from build123d import *

# Parameters (mm, degrees)
SKETCH1_R           = 5.78131598
BOSS_EXTRUDE1_DEPTH = 12.7
SKETCH2_W           = 12.7
SKETCH2_H           = 6.35
CUT_EXTRUDE1_DEPTH  = 33.528


with BuildPart() as part:
    # Sketch1 → Boss-Extrude1 (new body)
    with BuildSketch(Plane(origin=(0, 0, 0), x_dir=(1, 0, 0), z_dir=(0, 1, 0))):
        with BuildLine():
            Line((-36.7158591, 9.525), (-62.1158591, 9.525))
            Line((-62.1158591, 9.525), (-62.1158591, 28.575))
            ThreePointArc((-62.1158591, 28.575), (-49.4158591, 41.275), (-36.7158591, 28.575))
            Line((-36.7158591, 28.575), (-36.7158591, 9.525))
        make_face()
        with Locations(Location((-49.4158591, 28.575, 0), (0, 0, 270))):
            Circle(SKETCH1_R, mode=Mode.SUBTRACT)
    extrude(amount=BOSS_EXTRUDE1_DEPTH)

    # Sketch2 → Cut-Extrude1 (cut)
    with BuildSketch(Plane(origin=(-36.7158591, 0, 0), x_dir=(0, 0, -1), z_dir=(1, 0, 0))):
        with Locations((34.925, 6.35)):
            Rectangle(SKETCH2_W, SKETCH2_H)
        Polygon((28.575, 9.525), (12.7, 9.525), (12.7, 6.35), (12.7, 3.175), (28.575, 3.175), align=None)
    extrude(amount=-CUT_EXTRUDE1_DEPTH, mode=Mode.SUBTRACT)


solid = part.part
Part model, mm, in its own coordinate system. A direction names the side the tool comes from. Give positions to 0.01 mm unless a question says otherwise; leave off trailing zeros. Loops run counter-clockwise (first coordinate to the right, second up) from the corner with the lowest first, then second, coordinate; pieces in that order, holes last. Notation, with made-up numbers: (28, 66.5) -> (72, 66.5) arc R21 cw to (72, 80.5) -> close; hole circle Ø6 at (-6.5, 74.5). An arc over 180 degrees is marked (long way). Write each question's results on one line, items separated by ' | '. Start each with the question number.
Q1. Pull direction X, two halves, no side cores. Call faces 1 (the face through (-47.68, 1.57, -23.06)), 2 (the face through (-62.116, 2, -17)), 3 (the face through (-49, 6, -12.7)): +X half, -X half, draft (parallel to the pull), parting line (faces both ways), or undercut.
Q2. Band-saw the part on C-C on x = -53. List the corners of the cut face in (y, z) (3 decimals).
Q3. Wall check: L1, parallel to Y at x = -40.75, z = -23.5 (3 decimals); L2, parallel to Z at x = -38.5, y = 5.75 (3 decimals); L3, parallel to X at y = 10.5, z = -32.5. Give the ranges that are in metal, low to high.
Q4. Band-saw the part on D-D on y = 11. List the corners of the cut face in (x, z) (3 decimals), plus the area to 3 significant figures.
Q5. Band-saw the part on B-B on z = -24. List the corners of the cut face in (x, y) (3 decimals), plus the area to 3 significant figures.
Q6. Pin check, flat tips, straight feed: P1, Ø10, axis at x = -57, z = -24.5, coming from the -Y side; P2, Ø1.5, axis at x = -49, y = 6, coming from the -Z side; P3, Ø2, axis at y = 6, z = -19, coming from the +X side; P4, Ø2, axis at y = 1.5, z = -34.5, coming from the -X side. Stop position of each tip, or through.
Q7. Band-saw the part on A-A on z = -18.5. List the corners of the cut face in (x, y) (3 decimals), plus the area to 3 significant figures.
Q8. Which spindle directions (+Z, -Z, +X, -X, +Y, -Y) get a long thin tool onto all of the face, cutting with end or side? Do faces 4 (the face through (-49, 9.525, -21)), 5 (the face through (-49.7, 11.09, -41.27)). Say none if no direction does.
Results are:
1) face 1: undercut | face 2: -X half | face 3: draft
2) outline: (0, -40.759) -> (3.175, -40.759) -> (3.175, -33.111) -> (0, -33.111) -> close; (0, -24.039) -> (3.175, -24.039) -> (3.175, -12.7) -> (9.525, -12.7) -> (9.525, -24.039) -> (12.7, -24.039) -> (12.7, -9.525) -> (0, -9.525) -> close; (9.525, -40.759) -> (12.7, -40.759) -> (12.7, -33.111) -> (9.525, -33.111) -> close
3) L1: y = 0 to 3.175, 9.525 to 12.7 | L2: z = -12.7 to -9.525 | L3: x = -61.49 to -53.66, -45.17 to -37.34
4) outline: (-62.116, -28.575) arc R12.7 ccw to (-36.716, -28.575) -> (-36.716, -9.525) -> (-62.116, -9.525) -> close; hole circle Ø11.563 at (-49.416, -28.575) | area: 632 mm²
5) outline: (-62.116, 0) -> (-52.95, 0) -> (-52.95, 3.175) -> (-62.116, 3.175) -> close; (-62.116, 9.525) -> (-52.95, 9.525) -> (-52.95, 12.7) -> (-62.116, 12.7) -> close; (-45.881, 0) -> (-36.716, 0) -> (-36.716, 3.175) -> (-45.881, 3.175) -> close; (-45.881, 9.525) -> (-36.716, 9.525) -> (-36.716, 12.7) -> (-45.881, 12.7) -> close | area: 116 mm²
6) P1: stops at y = 0 | P2: stops at z = -12.7 | P3: passes through | P4: stops at x = -61.12
7) outline: (-62.116, 0) -> (-36.716, 0) -> (-36.716, 3.175) -> (-62.116, 3.175) -> close; (-62.116, 9.525) -> (-36.716, 9.525) -> (-36.716, 12.7) -> (-62.116, 12.7) -> close | area: 161 mm²
8) face 4: -Z, +X, -X | face 5: -Z, +Y, -Y
